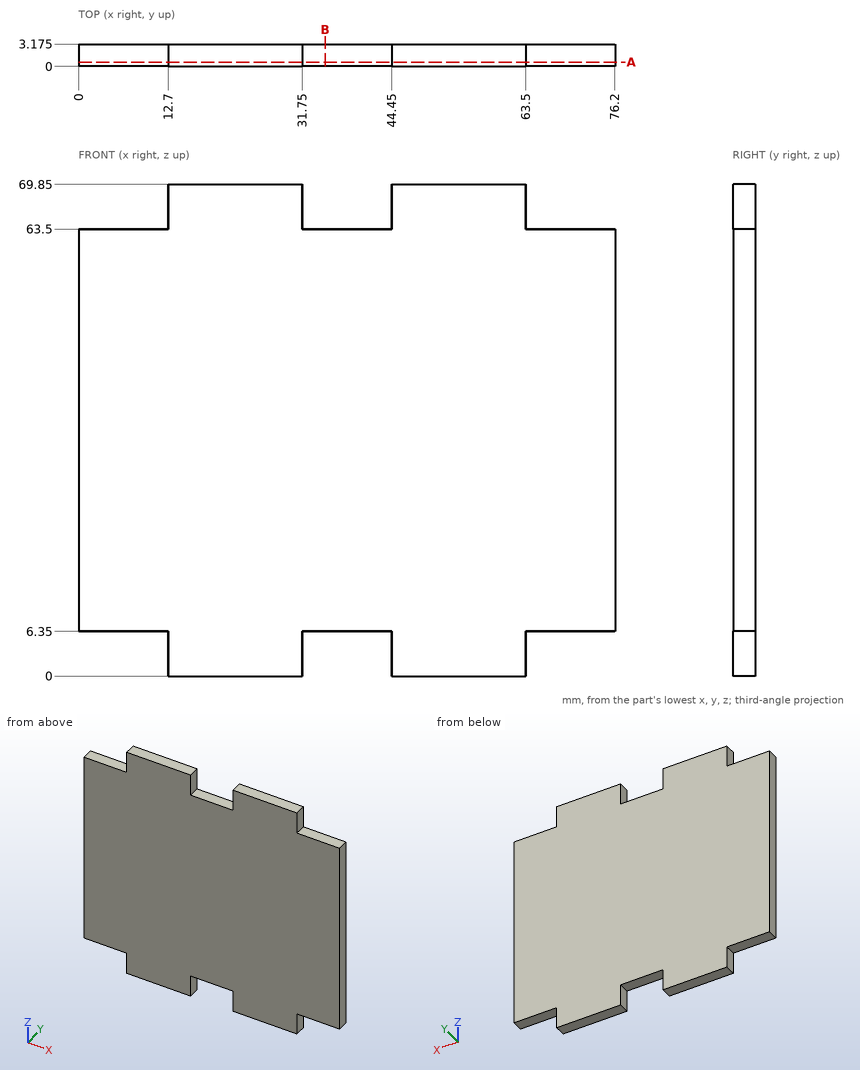
Design review of the part shown in the three views and the two pictorial views. Dimensions are in mm from the part's minimum x, y and z. Coordinates: 2 decimals unless noted, no trailing zeros. Order: outer loops, then holes, each group sorted by start corner. A loop starts at its lowest first (then second) coordinate and runs counter-clockwise, first axis right, second up.
1) Take a section at A-A, the plane y = 0.6. Give the boundary of the cut face in (x, z), and give its area (3 significant figures).
2) Clearance check with flat-ended pins moving along their axes: pin 1 (1.6 mm diameter, centred on y = 2, z = 4.5, fed in from +X); pin 2 (1 mm diameter, centred on x = 41, y = 2, fed in from -Z); pin 3 (1.6 mm diameter, centred on y = 1.5, z = 3.5, fed in from -X); pin 4 (5 mm diameter, centred on x = 62.5, z = 25, fed in from -Y). State where each tip first meets the part, or that it passes through.
3) Wall thickness on line 1 along Z through (x, y) = (6, 1.1); line 2 along X through (y, z) = (2.7, 65): over which ranges is each line inside the solid? List them lowest first.
4) Take a section at B-B, the plane x = 35. Give the boundary of the cut face in (y, z) (3 decimals).
Returned:
1. outline: (0, 6.35) - (12.7, 6.35) - (12.7, 0) - (31.75, 0) - (31.75, 6.35) - (44.45, 6.35) - (44.45, 0) - (63.5, 0) - (63.5, 6.35) - (76.2, 6.35) - (76.2, 63.5) - (63.5, 63.5) - (63.5, 69.85) - (44.45, 69.85) - (44.45, 63.5) - (31.75, 63.5) - (31.75, 69.85) - (12.7, 69.85) - (12.7, 63.5) - (0, 63.5) - close
1. area: 4,840 mm2
2. pin 1: stops at x = 63.5
2. pin 2: stops at z = 6.35
2. pin 3: stops at x = 12.7
2. pin 4: stops at y = 0
3. line 1: z = 6.35 to 63.5
3. line 2: x = 12.7 to 31.75, 44.45 to 63.5
4. outline: (0, 6.35) - (3.175, 6.35) - (3.175, 63.5) - (0, 63.5) - close
